Build history of the part. All positions in model axes, mm. Round coordinates to 2 decimals unless told otherwise and drop trailing zeros. Write each loop counter-clockwise with the first axis right and the second up, starting at its lowest first coordinate (ties: lowest second). Pieces come first, ordered by that corner, then holes. Notation, with made-up numbers: M 39.25,33 L 66.25,33 A25 cw 66.25,69 Z; hole C 60.25,71 d6. An arc over 180 degrees is marked long. Write item = value, one per line. Start each with the question number.
Q1. Probe L1, parallel to X at y = 11.5, z = 14.5; L2, parallel to X at y = 7.5, z = 15.25; L3, parallel to Y at x = -12, z = 22. List the from-to ranges inside material, lowest first.
Q2. Pull direction Y, two halves, no side cores. Call faces 1 (the cylindrical face through (0.334, 15.196, 15.707)), 2 (the flat face through (-31, 12, 16)): released by +Y, released by -Y, zero draft, split by the parting line, or undercut.
Q3. Drop flat-ended pins along their axis: P1, Ø4, axis at x = 20.5, y = 8, coming from the +Z side; P2, Ø2, axis at x = -19.5, z = 22.5, coming from the -Y side; P3, Ø5, axis at y = 4, z = 15, coming from the -X side; P4, Ø4, axis at x = 7, z = 6.5, coming from the +Y side. Give the stop position or say it passes through.
Q4. Band-saw the part on A-A on x = 0. Write the cut outline in (y, z), plus the area to 3 significant figures.
```python
from build123d import *

# Parameters (mm, degrees)
REARWINGBASE_DEPTH   = 26
CLEARENCE_DEPTH      = 26
CLEARENCE_DEPTH_BACK = 26
REARWING_DEPTH       = 31
REARWING_DEPTH_BACK  = 31
CLEARENCE2_START     = -26
SKETCH10_R           = 14.2
CLEARENCE2_DEPTH     = 26


with BuildPart() as part:
    # Sketch4 → RearWingBase (new body)
    with BuildSketch(Plane.XY):
        with BuildLine():
            Line((-15.2, 0), (-14.2, 0))
            ThreePointArc((-14.2, 0), (0, 14.2), (14.2, 0))
            Line((14.2, 0), (15.2, 0))
            ThreePointArc((15.2, 0), (0, 15.2), (-15.2, 0))
        make_face()
    extrude(amount=REARWINGBASE_DEPTH)

    # Sketch6 → Clearence (cut, two sides: drawn at the far end of the back side and taken through both)
    with BuildSketch(Plane(origin=(0, 0, 0), x_dir=(0, 0, -1), z_dir=(1, 0, 0)).offset(-CLEARENCE_DEPTH_BACK)):
        with BuildLine():
            Line((0.002719324, 13.829604024), (0.002719324, 15.197805772))
            Line((0.002719324, 15.197805772), (5.416214623, 15.197805772))
            Line((5.416214623, 15.197805772), (5.416214623, -5.766909468))
            Line((5.416214623, -5.766909468), (-19.095204108, -5.766909468))
            add(Edge.make_bspline(
                [(-19.095204108, -5.766909468), (-17.667809088, -0.279268361), (-14.718368277, 4.473703473), (-9.161470645, 11.138949331), (-3.695889294, 13.315625567), (0.002719324, 13.829604024)],
                knots=[0, 0, 0, 0, 0.423900901, 0.523900901, 1, 1, 1, 1], degree=3))
        make_face()
    extrude(amount=CLEARENCE_DEPTH + CLEARENCE_DEPTH_BACK, mode=Mode.SUBTRACT)

    # Sketch7 → RearWing (add, two sides: drawn at the far end of the back side and taken through both)
    with BuildSketch(Plane(origin=(0, 0, 0), x_dir=(0, 0, -1), z_dir=(1, 0, 0)).offset(-REARWING_DEPTH_BACK)):
        with BuildLine():
            add(Edge.make_bspline(
                [(-23.31622835, 11.867098708), (-21.717058728, 12.055213608), (-17.709554302, 12.634200705), (-16.496163082, 12.809494118), (-14.984125288, 12.779042837)],
                knots=[0, 0, 0, 0, 0.450119824, 1, 1, 1, 1], degree=3))
            add(Edge.make_bspline(
                [(-14.984125288, 12.779042837), (-11.626410325, 12.668851451), (-11.573129472, 11.081257235), (-14.968657337, 10.907420766)],
                knots=[0, 0, 0, 0, 1, 1, 1, 1], degree=3))
            add(Edge.make_bspline(
                [(-23.31622835, 11.867098708), (-19.356721106, 11.506371016), (-17.965634836, 10.821641279), (-14.968657337, 10.907420766)],
                knots=[0, 0, 0, 0, 1, 1, 1, 1], degree=3))
        make_face()
    extrude(amount=REARWING_DEPTH + REARWING_DEPTH_BACK)

    # Sketch10 → Clearence2 (cut)
    with BuildSketch(Plane.XY.offset(26).offset(CLEARENCE2_START)):
        Circle(SKETCH10_R)
    extrude(amount=CLEARENCE2_DEPTH, mode=Mode.SUBTRACT)


solid = part.part
```
Conclusion:
q1.L1 = -31 to -8.33, 8.33 to 31
q1.L2 = -13.22 to -12.06, 12.06 to 13.22
q1.L3 = 7.59 to 9.33, 11.73 to 12.03
q2.face_1 = undercut
q2.face_2 = zero draft
q3.P1 = through
q3.P2 = 11.66
q3.P3 = -15.1
q3.P4 = 14.35
q4.outline = M 14.2,0 L 15.2,0 L 15.2,26 L 14.2,26 Z
q4.area = 26.0 mm^2
